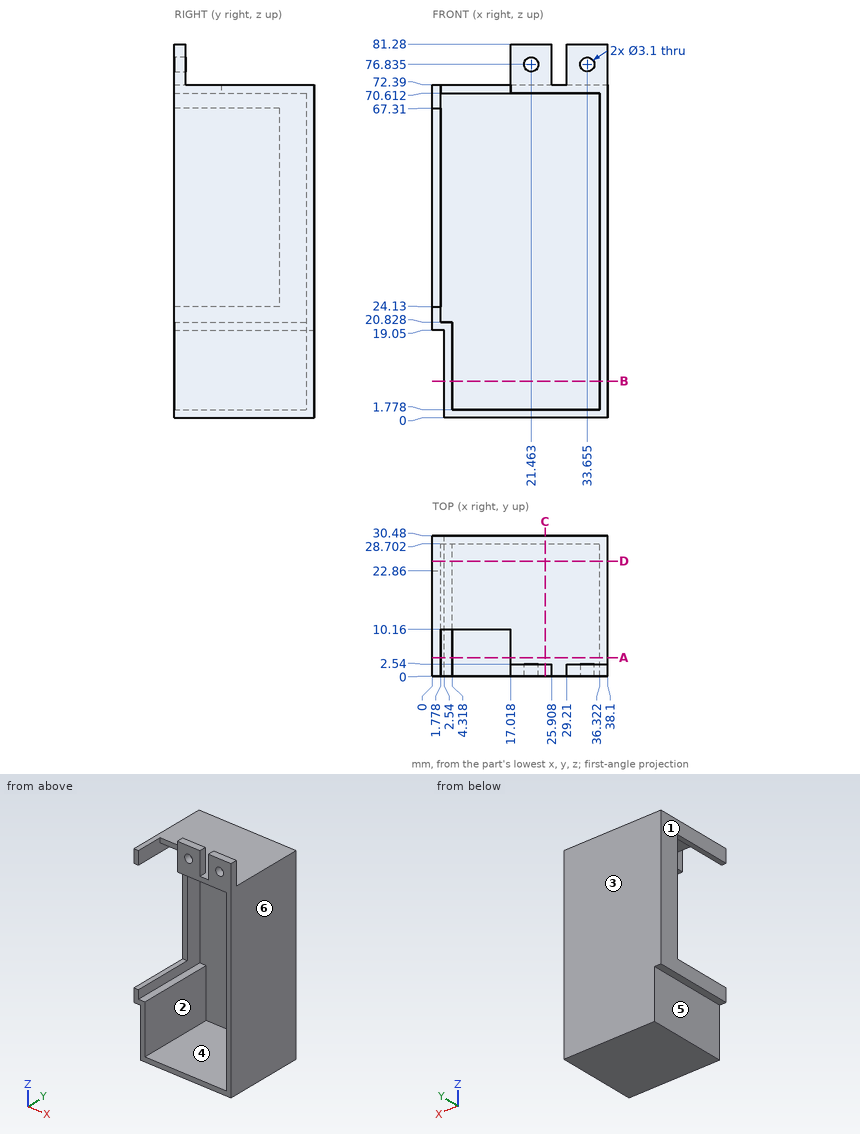
Verification items for this drawing (mm, ordinates from the low corner). A direction names the side the tool comes from. Coordinates: 2 decimals unless noted, no trailing zeros. Write each loop counter-clockwise with the first axis right and the second up, starting at its lowest first coordinate (ties: lowest second). Pieces come first, ordered by that corner, then holes. Notation, with made-up numbers: (77, 48) -> (108, 48) arc R18 cw to (108, 57) -> close; hole circle Ø11 at (42, 64). An arc over 180 degrees is marked (long way). One line per item, written item: value. Start each with the question number.
Q1. Mould release check, pull along X, two halves, no side actions. Record for the marked faces 1, 2 and 3: pulls with the +X half, pulls with the -X half, needs draft (parallel to the pull), parting line crosses it, or undercut.
Q2. Cross-section at C-C on x = 24.5. Enter the section's corners in (y, z).
Q3. Cross-section at A-A on y = 4. Enter the section's corners in (x, z).
Q4. Access from +Z, -Z, +X, -X, +Y, -Y to the whole of each face (thin tool, end or side, straight path). Record for the marked faces 4, 5 and 6.
Q5. Cross-section at D-D on y = 25. Enter the section's corners in (x, z), and give its area (3 significant figures).
Q6. Cross-section at B-B on z = 8. Enter the section's corners in (x, y).
Q7. Go/stop test with flat-tipped pins: P1, Ø2, axis at x = 1, z = 56, coming from the -Y side; P2, Ø0.5, axis at x = 1, y = 10, coming from the -Z side; P3, Ø17.5, axis at x = 21.5, z = 47.5, coming from the -Y side. Record where each tip stops, or that it passes through.
Q8. Thickness scan on L1, parallel to Z at x = 20, y = 15; L2, parallel to X at y = 8, z = 8.5; L3, parallel to X at y = 25.5, z = 59.5. Record the ranges inside material, lowest first. Write a range as from..to.
Checked values:
1. face 1: pulls with the -X half
1. face 2: undercut
1. face 3: needs draft
2. outline: (0, 0) -> (30.48, 0) -> (30.48, 72.39) -> (2.54, 72.39) -> (2.54, 81.28) -> (0, 81.28) -> (0, 70.61) -> (28.7, 70.61) -> (28.7, 1.78) -> (0, 1.78) -> close
3. outline: (0, 19.05) -> (2.54, 19.05) -> (2.54, 0) -> (38.1, 0) -> (38.1, 72.39) -> (17.02, 72.39) -> (17.02, 70.61) -> (36.32, 70.61) -> (36.32, 1.78) -> (4.32, 1.78) -> (4.32, 20.83) -> (1.78, 20.83) -> (1.78, 24.13) -> (0, 24.13) -> close; (0, 67.31) -> (1.78, 67.31) -> (1.78, 72.39) -> (0, 72.39) -> close
4. face 4: -Y
4. face 5: -Z, -X, +Y, -Y
4. face 6: +Z, -Z, +X, +Y, -Y
5. outline: (0, 19.05) -> (2.54, 19.05) -> (2.54, 0) -> (38.1, 0) -> (38.1, 72.39) -> (0, 72.39) -> close; hole (1.78, 20.83) -> (4.32, 20.83) -> (4.32, 1.78) -> (36.32, 1.78) -> (36.32, 70.61) -> (1.78, 70.61) -> close
5. area: 380 mm²
6. outline: (2.54, 0) -> (4.32, 0) -> (4.32, 28.7) -> (36.32, 28.7) -> (36.32, 0) -> (38.1, 0) -> (38.1, 30.48) -> (2.54, 30.48) -> close
7. P1: stops at y = 22.86
7. P2: stops at z = 19.05
7. P3: stops at y = 28.7
8. L1: z = 0..1.78, 70.61..72.39
8. L2: x = 2.54..4.32, 36.32..38.1
8. L3: x = 0..1.78, 36.32..38.1
